Autodesk Inventor part; units mm, degrees
ref_plane "Work Plane1" through (0, 0, 0) normal (-0.5, 0, -0.866) x (0, 1, 0)
ref_plane "XZ Plane" through (0, 0, 0) normal (0, 1, 0) x (-1, 0, 0)
ref_plane "XY Plane" through (0, 0, 0) normal (0, 0, 1) x (1, 0, 0)
sketch "Sketch2" plane through (0, 0, 0) normal (0, 1, 0) x (-1, 0, 0)
  line L0 (-20, -7.5) -> (-20, 7.5)
  line L1 (-20, 7.5) -> (20, 7.5)
  line L2 (20, 7.5) -> (20, -7.5)
  arc A0 (-2.3, -7.5) -> (2.3, -7.5) centre (0, -11.8267) ccw
  line L3 (20, -7.5) -> (2.3, -7.5)
  line L4 (-2.3, -7.5) -> (-20, -7.5)
  point P0 (0, 0)
  point P1 (0, -7.5)
  point P2 (-20, 0)
  point P3 (0, -16.7267)
  dimension "d1" = 40
  dimension "d3" = 15
  dimension "d5" = 4.6
  dimension "d6" = 4.9
extrude "Extrusion1" add sketch "Sketch2" along normal mid plane 3
ref_plane "Work Plane1" through (0, 0, 0) normal (-0.5, 0, -0.866) x (0, 1, 0)
sketch "Sketch3" plane through (0, 0, 0) normal (-0.5, 0, -0.866) x (0, 1, 0)
  line L0 (1.5, 1.7581) -> (1.5, -13.5705)
  line L1 (8.5, -3) -> (1.5, -3)
  line L2 (1.5, -3) -> (1.5, 5)
  line L3 (1.5, 5) -> (8.5, 5)
  line L4 (8.5, 5) -> (8.5, -3)
  line L5 (8.5, 1) -> (1.5, 1) construction
  line L6 (6.35, 7) -> (7.35, 9) construction
  line L7 (7, 7) -> (8, 9) construction
  line L8 (8, 9) -> (7.35, 9) construction
  line L9 (7, 7) -> (6.35, 7)
  line L10 (8.5, -3) -> (11.65, -3)
  line L11 (11.65, -3) -> (11.65, 5)
  line L12 (11.65, 5) -> (8.5, 5)
  line L13 (7, 7) -> (6, 5)
  line L14 (6.35, 7) -> (5.35, 5)
  line L15 (8.5, -3) -> (12.65, -3)
  line L16 (12.65, -3) -> (12.65, 5)
  line L17 (12.65, 5) -> (8.5, 5)
  point P0 (0, 0)
  point P1 (5, 1)
  point P2 (1.5, -3)
  dimension "d10" = 8
  dimension "d11" = 7
  dimension "d15" = 4
  dimension "d16" = 1
  dimension "d17" = 2.3
  dimension "d18" = 6.3
  dimension "d19" = 6.3
  dimension "d22" = 8.3
  dimension "d25" = 1
extrude "Extrusion2" add sketch "Sketch3" along normal mid plane 10 contours L2 L3 L4 L1 L0
revolve "Revolution1" cut sketch "Sketch3" angle 360 about axis through (4.3301, 8.5, -2.5) along (-0.866, 0, 0.5) contours L4 L12 L11 L10
revolve "Revolution2" add sketch "Sketch3" angle 360 about axis through (4.3301, 8.5, -2.5) along (-0.866, 0, 0.5) contours L11 L17 L16 L15
equation "\"d19\" = d18"
properties part number "Nozzle Fixer"
Work out the finished part from the listing and answer in its coordinate system (mm). A direction names the side the tool comes from. Give positions to 0.01 mm unless a question says otherwise; leave off trailing zeros. Loops run counter-clockwise (first coordinate to the right, second up) from the corner with the lowest first, then second, coordinate; pieces in that order, holes last. Notation, with made-up numbers: (12, -20) - (27, -20) arc R31 ccw to (27, 8) - close; hole circle Ø7 at (18, 44.5). An arc over 180 degrees is marked (long way). Answer in a Markdown table with one row per item. Add a question column.
Q1. The part is cut by section A-A (y = 10.5). Determine the outline of the cut face in (x, z).
Q2. A tool of negligible diameter and unlimited length cuts with its end or side. For faces 4 (the flat face through (4.295, 4.519, -2.561)), 5 (the flat face through (-2.633, 4.519, 1.439)), 6 (the flat face through (3.415, 4.951, 3.802)), 7 (the flat face through (-1.585, 4.951, -4.858)), from which of +Z, -Z, +X, -X, +Y, -Y can it reach the whole face along a straight path? Write none if from no direction.
Q3. Each of these flat-tipped pins is pushed along its axis until it touches: P1, Ø2.5, axis at x = 4.5, z = 4.5, coming from the +Y side; P2, Ø4, axis at y = 0, z = -13, coming from the -X side; P3, Ø1.5, axis at x = 14.5, y = 0, coming from the -Z side; P4, Ø8, axis at x = -12, y = 5, coming from the +Z side. Where does it stop, or does it pass through?
Q4. Determine the mould class of faces 1 (the flat face through (20, 0, 0)), 2 (the cylindrical face through (0.31, 11.41, -1.57)), 3 (the cylindrical face through (0.87, 12.65, -0.61)) for opening direction X: released by +X, released by -X, zero draft, split by the parting line, or undercut.
Q5. Consider line 1 along Z through (x, y) = (-15, -0.75); line 2 along Z through (x, y) = (1, 11.25); line 3 along Y through (x, z) = (-5, -4.5). Determine where each line is inside the solid, lowest interval first.
Q6. The part is cut by section C-C (y = 2). Determine the outline of the cut face in (x, z), and give its area (3 significant figures).
Q7. The part is cut by section B-B (x = 8.5). Determine the outline of the cut face in (y, z), and give its area (3 significant figures).
Q8. The part is cut by section D-D (y = 7.25). Determine the outline of the cut face in (x, z).
Solution:
| question | item | result |
|---|---|---|
| 1 | outline | (-4.42, -1.65) - (2.51, -5.65) - (3.11, -4.61) - (-3.81, -0.61) - close; (-1.38, 3.61) - (5.55, -0.39) - (6.15, 0.65) - (-0.78, 4.65) - close |
| 2 | face 4 | -Z, +X, +Y |
| 2 | face 5 | +Z, -X, +Y |
| 2 | face 6 | +Z, +X, +Y |
| 2 | face 7 | -Z, -X, +Y |
| 3 | P1 | stops at y = 8.5 |
| 3 | P2 | stops at x = -4.9 |
| 3 | P3 | stops at z = -7.5 |
| 3 | P4 | stops at z = 7.5 |
| 4 | face 1 | released by +X |
| 4 | face 2 | undercut |
| 4 | face 3 | split by the parting line |
| 5 | line 1 | z = -7.5 to 7.5 |
| 5 | line 2 | z = -4.17 to -2.35, 1.2 to 3.01 |
| 5 | line 3 | y = -1.5 to 1.5 |
| 6 | outline | (-5.1, -2.83) - (1.83, -6.83) - (6.83, 1.83) - (-0.1, 5.83) - close |
| 6 | area | 80.0 mm² |
| 7 | outline | (-1.5, -7.5) - (1.5, -7.5) - (1.5, 7.5) - (-1.5, 7.5) - close |
| 7 | area | 45.0 mm² |
| 8 | outline | (-5.1, -2.83) - (1.83, -6.83) - (2.88, -5) - (-4.04, -1) - close; (-1.15, 4) - (5.78, 0) - (6.83, 1.83) - (-0.1, 5.83) - close |
